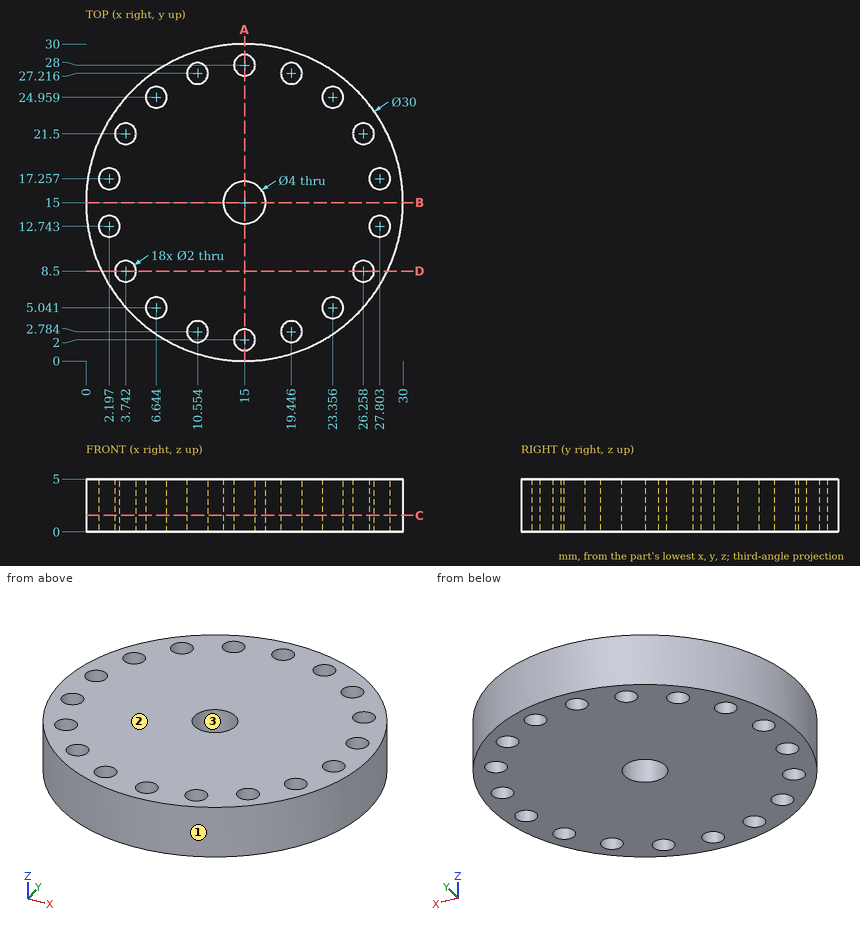
For this review, use the dimensioned drawing (mm, ordinates from the lowest corner) and the shaded views. Give positions to 0.01 mm unless a question says otherwise; leave off trailing zeros. Order: outer loops, then holes, each group sorted by start corner. A loop starts at its lowest first (then second) coordinate and runs counter-clockwise, first axis right, second up. Notation, with made-up numbers: (69.25, 40) - (119.25, 40) arc R17 ccw to (119.25, 62) - close; hole circle Ø8 at (78, 76). An arc over 180 degrees is marked (long way). Write item = value, one per line. Start each with the question number.
Q1. We need section C-C on z = 1.55. State how many separate pieces and enclosed holes the cut face has, plus the area to 3 significant figures.
Q2. We need section B-B on y = 15. State the section outline as (x, z) points, plus the area to 3 significant figures.
Q3. We need section D-D on y = 8.5. State the section outline as (x, z) points.
Q4. Clearance check with flat-ended pins moving along their axes: pin 1 Ø1.5 at (y, z) = (20.5, 2.5) entering from -X; pin 2 Ø1.5 at (x, z) = (5, 2) entering from +Y. State where each tip first meets the part, or that it passes through.
Q5. Mouldability with a two-part tool opening along X and no side actions: class the marked faces 1, 2 and 3 as released by +X, released by -X, zero draft, split by the parting line, or undercut.
Q6. To check wall thickness, follow L1, parallel to Y at x = 15, z = 2.45; L2, parallel to X at y = 26.75, z = 1.5 (1 decimal); L3, parallel to Y at x = 1.5, z = 4.85 (1 decimal). State the ranges of each line that lie inside material, in increasing order. Write a range as from..to.
Q7. We need section A-A on x = 15. State the section outline as (y, z) points.
Working result:
q1.separate_pieces = 1
q1.enclosed_holes = 19
q1.area = 638 mm²
q2.outline = (0, 0) - (13, 0) - (13, 5) - (0, 5) - close; (17, 0) - (30, 0) - (30, 5) - (17, 5) - close
q2.area = 130 mm²
q3.outline = (1.48, 0) - (2.74, 0) - (2.74, 5) - (1.48, 5) - close; (4.74, 0) - (25.26, 0) - (25.26, 5) - (4.74, 5) - close; (27.26, 0) - (28.52, 0) - (28.52, 5) - (27.26, 5) - close
q4.pin_1 = 0.77
q4.pin_2 = 26.81
q5.face_1 = split by the parting line
q5.face_2 = zero draft
q5.face_3 = undercut
q6.L1 = 0..1, 3..13, 17..27, 29..30
q6.L2 = 5.7..9.7, 11.4..18.6, 20.3..24.3
q6.L3 = 8.5..12, 13.5..16.5, 18..21.5
q7.outline = (0, 0) - (1, 0) - (1, 5) - (0, 5) - close; (3, 0) - (13, 0) - (13, 5) - (3, 5) - close; (17, 0) - (27, 0) - (27, 5) - (17, 5) - close; (29, 0) - (30, 0) - (30, 5) - (29, 5) - close
